CAD build for the part. Positions are in the model's coordinates, mm. Face numbers are marked on the shaded views. Give positions to 0.01 mm unless a question says otherwise; leave off trailing zeros. Loops run counter-clockwise (first coordinate to the right, second up) from the corner with the lowest first, then second, coordinate; pieces in that order, holes last.
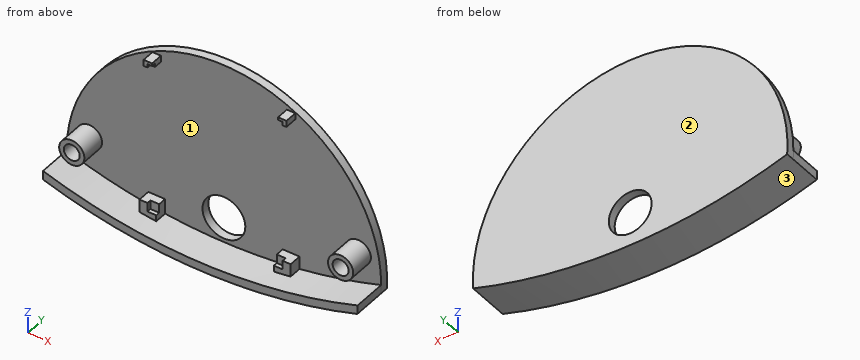
```python
from build123d import *
from build123d.topology import SkipClean

# Parameters (mm, degrees)
SKETCH_1_R      = 5.1
EXTRUDE_1_DEPTH = 2
EXTRUDE_START   = 8
EXTRUDE_2_DEPTH = 8
SKETCH_3_R      = 3
SKETCH_3_R_2    = 1.9
EXTRUDE_3_DEPTH = 6
SKETCH_4_W      = 4
SKETCH_4_H      = 4
SKETCH_4_W_2    = 2
SKETCH_4_H_2    = 1.5
EXTRUDE_4_DEPTH = 2
EXTRUDE_5_DEPTH = 1


with BuildPart() as part:
    # 草图1 → 凸台-拉伸1 (new body)
    with BuildSketch(Plane(origin=(0, 0, 0), x_dir=(1, 0, 0), z_dir=(0, 1, 0))):
        with BuildLine():
            ThreePointArc((-37.388863526, 2.139014778), (0, -37.45), (37.388863526, 2.139014778))
            ThreePointArc((37.388863526, 2.139014778), (0, 8), (-37.388863526, 2.139014778))
        make_face()
        with Locations(Location((0, 0, 0), (0, 0, 270))):
            Circle(SKETCH_1_R, mode=Mode.SUBTRACT)
    extrude(amount=EXTRUDE_1_DEPTH)

    # 草图2 → 凸台-拉伸2 (add)
    with SkipClean():  # the faces are left unmerged after this step: merging them gives an invalid solid
        with BuildSketch(Plane.XZ.offset(EXTRUDE_START)):
            with BuildLine():
                ThreePointArc((37.388863526, -2.139014778), (37.434477455, -1.078145477), (37.449996405, -0.016409414))
                ThreePointArc((37.449996405, -0.016409414), (0, -6), (-37.449996405, -0.016409414))
                ThreePointArc((-37.449996405, -0.016409414), (-37.434477455, -1.078145477), (-37.388863526, -2.139014778))
                ThreePointArc((-37.388863526, -2.139014778), (0, -8), (37.388863526, -2.139014778))
            make_face()
        extrude(amount=-EXTRUDE_2_DEPTH)

    # 草图3 → 凸台-拉伸3 (add)
    # profile 1 of 2: a face of its own
    with SkipClean():  # the faces are left unmerged after this step: merging them gives an invalid solid
        with BuildSketch(Plane.XZ):
            with Locations(Location((-32.006251973, 5.643565774, 0), (0, 0, 270))):
                Circle(SKETCH_3_R)
            with Locations(Location((-32.006251973, 5.643565774, 0), (0, 0, 270))):
                Circle(SKETCH_3_R_2, mode=Mode.SUBTRACT)
        # profile 2 of 2: a face of its own
        with BuildSketch(Plane.XZ):
            with Locations(Location((32.006251973, 5.643565774, 0), (0, 0, 270))):
                Circle(SKETCH_3_R)
            with Locations(Location((32.006251973, 5.643565774, 0), (0, 0, 270))):
                Circle(SKETCH_3_R_2, mode=Mode.SUBTRACT)
        extrude(amount=EXTRUDE_3_DEPTH)

    # 草图4 → 凸台-拉伸4 (add)
    with SkipClean():  # the faces are left unmerged after this step: merging them gives an invalid solid
        with BuildSketch(Plane.XZ):
            with Locations((16, -3.6)):
                Rectangle(SKETCH_4_W, SKETCH_4_H)
            with Locations((-16, -3.6)):
                Rectangle(SKETCH_4_W, SKETCH_4_H)
            with Locations((16, 32.4)):
                Rectangle(SKETCH_4_W_2, SKETCH_4_H_2)
            with Locations((-16, 32.4)):
                Rectangle(SKETCH_4_W_2, SKETCH_4_H_2)
        extrude(amount=EXTRUDE_4_DEPTH)

    # 草图5 → 凸台-拉伸5 (add)
    with SkipClean():  # the faces are left unmerged after this step: merging them gives an invalid solid
        with BuildSketch(Plane.XZ.offset(2)):
            Polygon((-16.1, 32.5), (-16.1, 31.65), (-17, 31.65), (-17, 33.15), (-15, 33.15), (-15, 32.5), align=None)
            Polygon((-16.1, -3.7), (-14, -3.7), (-14, -6.021052632), (-18, -6.021052632), (-18, -1.6), (-16.1, -1.6), align=None)
            Polygon((16.1, -3.7), (16.1, -1.6), (18, -1.6), (18, -5.6), (14, -5.6), (14, -3.7), align=None)
            Polygon((16.1, 32.5), (15, 32.5), (15, 33.15), (17, 33.15), (17, 31.65), (16.1, 31.65), align=None)
        extrude(amount=EXTRUDE_5_DEPTH)


solid = part.part
```
1. Drop flat-ended pins along their axis: pin 1 (0.9 mm diameter, centred on x = 16, y = -1.5, fed in from +Z); pin 2 (0.8 mm diameter, centred on y = -1.5, z = 32.5, fed in from -X); pin 3 (0.8 mm diameter, centred on x = -16.5, z = 32.5, fed in from -Y). Give the stop position or say it passes through.
Responses:
pin 1: stops at z = 33.15
pin 2: stops at x = -17
pin 3: stops at y = -3
2. Saw through at A-A, the plane x = 0. List the corners of the cut face in (y, z).
Responses:
outline: (-8, -8) - (2, -8) - (2, -5.1) - (0, -5.1) - (0, -6) - (-8, -6) - close; (0, 5.1) - (2, 5.1) - (2, 37.45) - (0, 37.45) - close
3. Saw through at B-B, the plane z = 1. List the corners of the cut face in (x, y).
Responses:
outline: (-37.44, 0) - (-5, 0) - (-5, 2) - (-37.44, 2) - close; (5, 0) - (37.44, 0) - (37.44, 2) - (5, 2) - close
4. Saw through at D-D, the plane z = 25.5. List the corners of the cut face in (x, y), and give its area (3 significant figures).
Responses:
outline: (-27.43, 0) - (27.43, 0) - (27.43, 2) - (-27.43, 2) - close
area: 110 mm2
5. Probe line 1 along Z through (x, y) = (1, -4.25); line 2 along X through (y, z) = (0.95, 0); line 3 along Y through (x, z) = (12, 31). List the from-to ranges inside material, lowest first.
Responses:
line 1: z = -8 to -6
line 2: x = -37.45 to -5.1, 5.1 to 37.45
line 3: y = 0 to 2
6. Saw through at C-C, the plane x = 20.5. List the corners of the cut face in (y, z), and give its area (3 significant figures).
Responses:
outline: (-8, -6.27) - (2, -6.27) - (2, 31.34) - (0, 31.34) - (0, -4.24) - (-8, -4.24) - close
area: 91.5 mm2
7. Pull direction Z, two halves, no side cores. Call the marked faces 1, 2 and 3: released by +Z, released by -Z, zero draft, split by the parting line, or undercut.
Responses:
face 1: undercut
face 2: zero draft
face 3: released by -Z
